from build123d import *

# Parameters (mm, degrees)
SKETCH1_W           = 20.8
SKETCH1_H           = 2.5
BOSS_EXTRUDE1_DEPTH = 8.35
SKETCH2_R           = 0.5
CUT_EXTRUDE1_DEPTH  = 3
SKETCH3_R           = 0.2
BOSS_EXTRUDE2_DEPTH = 3.2
LPATTERN1_COUNT     = 8
LPATTERN1_PITCH     = 2.54


with BuildPart() as part:
    # Sketch1 → Boss-Extrude1 (new body)
    with BuildSketch(Plane(origin=(0, 0, 0), x_dir=(1, 0, 0), z_dir=(0, 1, 0))):
        Rectangle(SKETCH1_W, SKETCH1_H)
    extrude(amount=BOSS_EXTRUDE1_DEPTH)

    # Sketch2 → Cut-Extrude1 (cut)
    with BuildSketch(Plane(origin=(0, 8.35, 0), x_dir=(1, 0, 0), z_dir=(0, 1, 0))):
        with Locations((-8.83, 0)):
            Circle(SKETCH2_R)
    cut_extrude1 = extrude(amount=-CUT_EXTRUDE1_DEPTH, mode=Mode.SUBTRACT)

    # Sketch3 → Boss-Extrude2 (add)
    with BuildSketch(Plane.XZ):
        with Locations((-8.83, 0)):
            Circle(SKETCH3_R)
    boss_extrude2 = extrude(amount=BOSS_EXTRUDE2_DEPTH)

    # LPattern1: Cut-Extrude1, Boss-Extrude2 ×8
    with Locations(*[(i * LPATTERN1_PITCH, 0, 0) for i in range(1, LPATTERN1_COUNT)]):
        add(cut_extrude1, mode=Mode.SUBTRACT)
        add(boss_extrude2)


solid = part.part
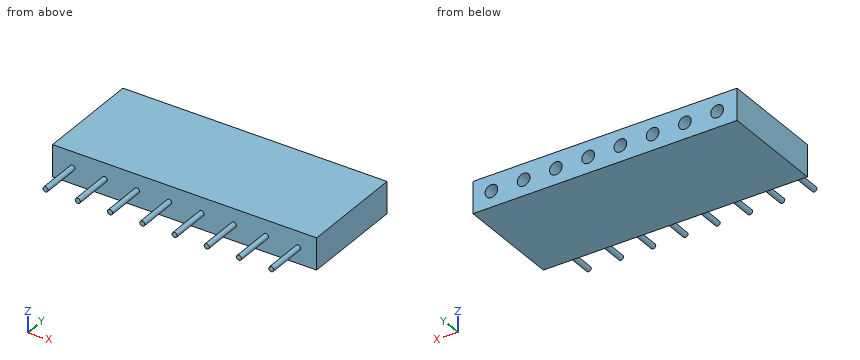
Geometry check sheet. Reference: the model listing, model coordinates, mm. Round coordinates to 2 decimals unless told otherwise and drop trailing zeros. Order: outer loops, then holes, each group sorted by start corner. A loop starts at its lowest first (then second) coordinate and runs counter-clockwise, first axis right, second up. Notation, with made-up numbers: M -33,70 L -29,70 A17 ccw -29,76 Z; hole C 21.25,-18.5 d9. An arc over 180 degrees is marked long. Write each question's results on one line, items separated by ' | '. Start each with the question number.
1. Cross-section at B-B on x = 8.95. Record the boundary of the cut face in (y, z), plus the area to 3 significant figures.
2. Material ranges on L1, parallel to Z at x = -6.29, y = 6.95; L2, parallel to Y at x = -2, z = 1; L3, parallel to Y at x = 9, z = 0.35, recorded low to high. Write a range as from..to.
3. Cross-section at D-D on z = 1. Record the boundary of the cut face in (x, y).
4. Cross-section at C-C on y = 6.25. Give the number of separate pieces and of enclosed holes in the cut face, plus the area to 3 significant figures.
5. Cross-section at A-A on y = -2.25. Record the boundary of the cut face in (x, z), plus the area to 3 significant figures.
Resolved:
1) outline: M -3.2,-0.2 L 0,-0.2 L 0,-1.25 L 8.35,-1.25 L 8.35,-0.5 L 5.35,-0.5 L 5.35,0.5 L 8.35,0.5 L 8.35,1.25 L 0,1.25 L 0,0.2 L -3.2,0.2 Z | area: 19.2 mm2
2) L1: -1.25..-0.5, 0.5..1.25 | L2: 0..8.35 | L3: 0..5.35
3) outline: M -10.4,0 L 10.4,0 L 10.4,8.35 L -10.4,8.35 Z
4) separate pieces: 1 | enclosed holes: 8 | area: 45.7 mm2
5) outline: C -8.83,0 d0.4; C -6.29,0 d0.4; C -3.75,0 d0.4; C -1.21,0 d0.4; C 1.33,0 d0.4; C 3.87,0 d0.4; C 6.41,0 d0.4; C 8.95,0 d0.4 | area: 1.01 mm2
